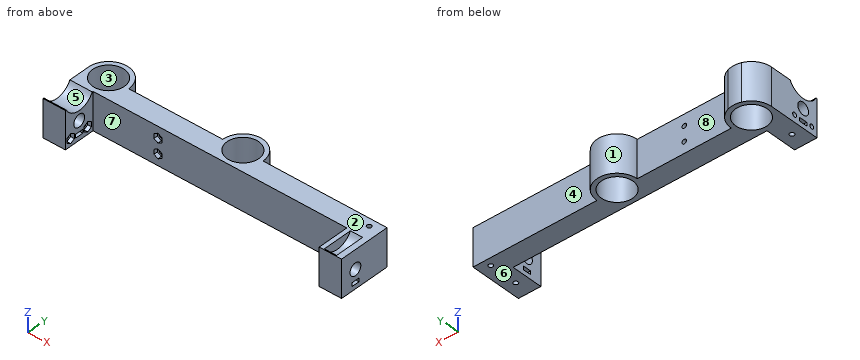
```python
from build123d import *

# Parameters (mm, degrees)
SKETCH007_R          = 10.6
PAD006_DEPTH         = 25
SKETCH016_R          = 4.1
SKETCH016_W          = 5.5
SKETCH016_H          = 2.4
POCKET008_DEPTH      = 58.501
POCKET008_DEPTH_BACK = 141.501
SKETCH024_R          = 11.1
SKETCH024_R_2        = 4.09
POCKET013_DEPTH      = 4.1
SKETCH025_R          = 1.5
POCKET014_DEPTH      = 13.501
POCKET014_DEPTH_BACK = 34.501
POCKET015_DEPTH      = 2.6
SKETCH027_R          = 1.5
POCKET016_DEPTH      = 12.5
SKETCH028_R          = 1.5
POCKET017_DEPTH      = 58.5010001
POCKET018_DEPTH      = 2.5
SKETCH032_R          = 1.5
POCKET019_DEPTH      = 0.001
POCKET019_DEPTH_BACK = 25.001
SKETCH033_R          = 11.1
POCKET020_DEPTH      = 58.5010001


with BuildPart() as part:
    # Sketch007 → Pad006 (new body)
    with BuildSketch(Plane.XY):
        with BuildLine():
            ThreePointArc((-31.5, 0), (-33.9772961575, 7.7942286341), (-40.5, 12.7279220614))
            ThreePointArc((-40.5, 12.7279220614), (-45, 13.5), (-49.5, 12.7279220614))
            ThreePointArc((-49.5, 12.7279220614), (-56.0227038425, 7.7942286341), (-58.5, 0))
            Line((-58.5, 0), (-58.5, -13.5))
            Line((-58.5, -17.2720779386), (-58.5, -13.5))
            Line((-58.5, -17.2720779386), (-58.5, -34.5))
            Line((-58.5, -34.5), (-43.5, -34.5))
            Line((-43.5, -34.5), (-43.5, -17.2720779386))
            Line((-43.5, -13.5), (-43.5, -17.2720779386))
            Line((-43.5, -13.5), (126.5, -13.5))
            Line((126.5, -34.5), (126.5, -13.5))
            Line((141.5, -34.5), (126.5, -34.5))
            Line((141.5, -13.5), (141.5, -34.5))
            Line((141.5, 0), (141.5, -13.5))
            Line((126.5, 0), (141.5, 0))
            Line((58.5, 0), (126.5, 0))
            ThreePointArc((58.5, 0), (45, 13.5), (31.5, 0))
            Line((-31.5, 0), (31.5, 0))
        make_face()
        with Locations((-45, 0)):
            Circle(SKETCH007_R, mode=Mode.SUBTRACT)
        with Locations((45, 0)):
            Circle(SKETCH007_R, mode=Mode.SUBTRACT)
    extrude(amount=PAD006_DEPTH)

    # Sketch016 → Pocket008 (cut, two sides)
    with BuildSketch(Plane.YZ) as pocket008_sk:
        with Locations((-24, 12.5)):
            Circle(SKETCH016_R)
        with Locations((-24, 4.2)):
            Rectangle(SKETCH016_W, SKETCH016_H)
    extrude(amount=-POCKET008_DEPTH, mode=Mode.SUBTRACT)
    extrude(pocket008_sk.sketch, amount=POCKET008_DEPTH_BACK, mode=Mode.SUBTRACT)

    # Sketch024 → Pocket013 (cut, symmetric)
    with BuildSketch(Plane.YZ.offset(133.5)):
        with Locations((-24, 30)):
            Circle(SKETCH024_R)
        with Locations((-24, 30)):
            Circle(SKETCH024_R_2, mode=Mode.SUBTRACT)
    extrude(amount=POCKET013_DEPTH, both=True, mode=Mode.SUBTRACT)

    # Sketch025 → Pocket014 (cut, two sides)
    with BuildSketch(Plane.XZ) as pocket014_sk:
        with Locations((0, 17.5)):
            Circle(SKETCH025_R)
        with Locations((0, 7.5)):
            Circle(SKETCH025_R)
    extrude(amount=-POCKET014_DEPTH, mode=Mode.SUBTRACT)
    extrude(pocket014_sk.sketch, amount=POCKET014_DEPTH_BACK, mode=Mode.SUBTRACT)

    # Sketch026 → Pocket015 (cut)
    with BuildSketch(Plane.XZ.offset(13.5)):
        Polygon((2.7, 19.0588457268), (0, 20.6176914536), (-2.7, 19.0588457268), (-2.7, 15.9411542732), (0, 14.3823085464), (2.7, 15.9411542732), align=None)
        Polygon((2.7, 9.0588457268), (0, 10.6176914536), (-2.7, 9.0588457268), (-2.7, 5.9411542732), (0, 4.3823085464), (2.7, 5.9411542732), align=None)
    extrude(amount=-POCKET015_DEPTH, mode=Mode.SUBTRACT)

    # Sketch027 → Pocket016 (cut)
    with BuildSketch(Plane.XY):
        with Locations((-51, -24)):
            Circle(SKETCH027_R)
        with Locations((134, -24)):
            Circle(SKETCH027_R)
    extrude(amount=POCKET016_DEPTH, mode=Mode.SUBTRACT)

    # Sketch028 → Pocket017 (cut, through all)
    with BuildSketch(Plane.YZ):
        with Locations((-30.5, 4.86)):
            Circle(SKETCH028_R)
        with Locations((-17.5, 4.86)):
            Circle(SKETCH028_R)
    extrude(amount=-POCKET017_DEPTH, mode=Mode.SUBTRACT)

    # Sketch029 → Pocket018 (cut)
    with BuildSketch(Plane.YZ.offset(-43.5)):
        Polygon((-27.7, 6.4765807537), (-30.5, 8.0931615075), (-33.3, 6.4765807537), (-33.3, 3.2434192463), (-30.5, 1.6268384925), (-27.7, 3.2434192463), align=None)
        Polygon((-20.3, 6.4765807537), (-20.3, 3.2434192463), (-17.5, 1.6268384925), (-14.7, 3.2434192463), (-14.7, 6.4765807537), (-17.5, 8.0931615075), align=None)
    extrude(amount=-POCKET018_DEPTH, mode=Mode.SUBTRACT)

    # Sketch032 → Pocket019 (cut, two sides)
    with BuildSketch(Plane.XY) as pocket019_sk:
        with Locations((134, -5)):
            Circle(SKETCH032_R)
    extrude(amount=-POCKET019_DEPTH, mode=Mode.SUBTRACT)
    extrude(pocket019_sk.sketch, amount=POCKET019_DEPTH_BACK, mode=Mode.SUBTRACT)

    # Sketch033 → Pocket020 (cut, through all)
    with BuildSketch(Plane.YZ):
        with Locations((-24, 30)):
            Circle(SKETCH033_R)
    extrude(amount=-POCKET020_DEPTH, mode=Mode.SUBTRACT)


with BuildPart() as part_1:
    # Body005 placement: moved
    add(part.part.moved(Location((0, 86, 0))))


solid = part_1.part
```
CAD build for the part. Positions are in the model's coordinates, mm. Face numbers are marked on the shaded views. A direction names the side the tool comes from. Round coordinates to 2 decimals unless told otherwise and drop trailing zeros. Loops run counter-clockwise (first coordinate to the right, second up) from the corner with the lowest first, then second, coordinate; pieces in that order, holes last. Notation, with made-up numbers: M 70,32.25 L 93,32.25 A22 cw 93,61.25 Z; hole C -24,-7.75 d1. An arc over 180 degrees is marked long. Use a Markdown table: item, result. Add a question column.
(1) Cut at B-B (y = 91). Give the cut face in (x, z).
(2) Cut at A-A (z = 12.5). Give the cut face in (x, y), and give its area (3 significant figures).
(3) Cut at D-D (z = 22.75). Give the cut face in (x, y).
(4) Which spindle directions (+Z, -Z, +X, -X, +Y, -Y) get a long thin tool onto all of the face, cutting with end or side? Do the marked faces 4, 5, 6, 7 and 8. Say none if no direction does.
(5) Flat gauge pins, fed straight in: pin 1 (2.5 mm diameter, centred on x = 0, z = 17.5, fed in from -Y); pin 2 (5 mm diameter, centred on x = 134, y = 62, fed in from +Z); pin 3 (3.5 mm diameter, centred on x = 0, z = 7.5, fed in from +Y); pin 4 (2.5 mm diameter, centred on x = -51, y = 62, fed in from +Z). Where does each tip first touch, or does it go through?
(6) Cut at C-C (x = 45). Give the cut face in (y, z), and give its area (3 significant figures).
(7) Pull direction Y, two halves, no side cores. Call the marked faces 1, 2 and 3: +Y half, -Y half, draft (parallel to the pull), parting line (faces both ways), or undercut.
(8) Drill centre lines: line 1 (Z direction, x = 0, y = 83); line 2 (X direction, y = 62, z = 6.85); line 3 (X direction, y = 72, z = 17.75). Where is each one in solid material? Low to high.
Geometry says:
| question | item | result |
|---|---|---|
| 1 | outline | M -57.54,0 L -54.35,0 L -54.35,25 L -57.54,25 Z; M -35.65,0 L -32.46,0 L -32.46,25 L -35.65,25 Z; M 32.46,0 L 35.65,0 L 35.65,25 L 32.46,25 Z; M 54.35,0 L 57.54,0 L 57.54,25 L 54.35,25 Z |
| 2 | outline | M -58.5,51.5 L -43.5,51.5 L -43.5,57.9 L -58.5,57.9 Z; M -58.5,66.1 L -43.5,66.1 L -43.5,72.5 L 126.5,72.5 L 126.5,66.1 L 141.5,66.1 L 141.5,86 L 58.5,86 A13.5 ccw 31.5,86 L -31.5,86 A13.5 ccw -58.5,86 Z; M 126.5,51.5 L 141.5,51.5 L 141.5,57.9 L 126.5,57.9 Z; hole C -45,86 d21.2; hole C 45,86 d21.2; hole C 134,81 d3 |
| 2 | area | 2,940 mm² |
| 3 | outline | M -58.5,51.5 L -43.5,51.5 L -43.5,53.59 L -58.5,53.59 Z; M -58.5,70.41 L -43.5,70.41 L -43.5,72.5 L 126.5,72.5 L 126.5,51.5 L 141.5,51.5 L 141.5,86 L 58.5,86 A13.5 ccw 31.5,86 L -31.5,86 A13.5 ccw -58.5,86 Z; hole C -45,86 d21.2; hole C 45,86 d21.2; hole M 129.4,53.59 L 137.6,53.59 L 137.6,70.41 L 129.4,70.41 Z; hole C 134,81 d3 |
| 4 | face 4 | +Z, -Z, +X, +Y |
| 4 | face 5 | +Z, -X |
| 4 | face 6 | -Z, +X, -X, +Y, -Y |
| 4 | face 7 | +Z, -Z, -Y |
| 4 | face 8 | +Z, -Z, +Y |
| 5 | pin 1 | passes through |
| 5 | pin 2 | stops at z = 19.19 |
| 5 | pin 3 | stops at y = 86 |
| 5 | pin 4 | stops at z = 18.97 |
| 6 | outline | M 72.5,0 L 75.4,0 L 75.4,25 L 72.5,25 Z; M 96.6,0 L 99.5,0 L 99.5,25 L 96.6,25 Z |
| 6 | area | 145 mm² |
| 7 | face 1 | +Y half |
| 7 | face 2 | draft |
| 7 | face 3 | undercut |
| 8 | line 1 | z = 0 to 6, 9 to 16, 19 to 25 |
| 8 | line 2 | x = -58.5 to -52.5, -49.5 to -43.5, 126.5 to 132.5, 135.5 to 141.5 |
| 8 | line 3 | x = -58.5 to -43.5, 126.5 to 141.5 |
